The drawing under review shows one solid part. Ordinate dimensions are in mm from its lowest x, y, z. A direction names the side the tool comes from. Coordinates: 2 decimals unless noted, no trailing zeros. Order: outer loops, then holes, each group sorted by start corner. A loop starts at its lowest first (then second) coordinate and runs counter-clockwise, first axis right, second up.
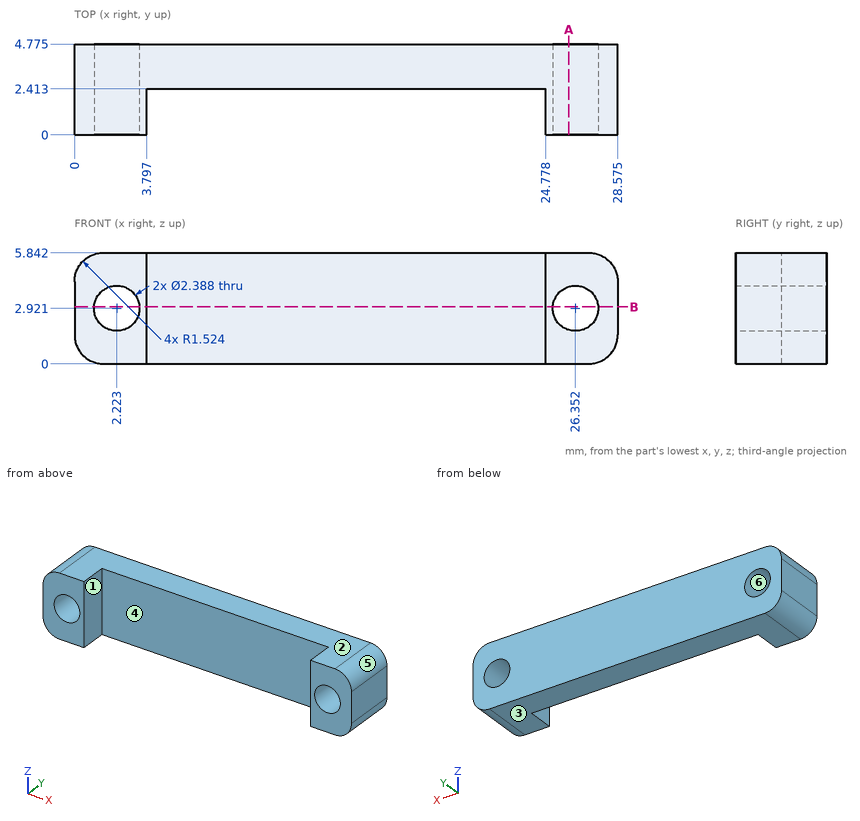
1. To check wall thickness, follow L1, parallel to X at y = 4, z = 2.85 (1 decimal); L2, parallel to X at y = 0.3, z = 1.45; L3, parallel to X at y = 3.4, z = 2 (1 decimal). State the ranges of each line that lie inside material, in increasing order.
Answer below:
L1: x = 0 to 1, 3.4 to 25.2, 27.5 to 28.6
L2: x = 0 to 3.8, 24.78 to 28.57
L3: x = 0 to 1.5, 3 to 25.6, 27.1 to 28.6
2. Machinability: for the marked faces 1 and 2, which of the approach directions +Z, -Z, +X, -X, +Y, -Y give a long, thin tool a straight path to every point of the face, cutting with its end or side? Answer none if there is none.
Answer below:
face 1: +Z, -Z, -Y
face 2: +Z, +X, -X, +Y, -Y
3. Clearance check with a flat-ended pin moving along its axis: pin 1 Ø1.4 at (x, z) = (26.35, 2.92) entering from -Y. State where the tip first meets the part, or that it passes through.
Answer below:
pin 1: passes through
4. The part is to be moulded in two halves that separate along Z. For the marked faces 3, 4, 5 and 6, say which applies: +Z half, -Z half, draft (parallel to the pull), parting line (faces both ways), or undercut.
Answer below:
face 3: -Z half
face 4: draft
face 5: +Z half
face 6: undercut
5. Take a section at A-A, the plane x = 26. Give the boundary of the cut face in (y, z) (1 decimal), plus the area to 3 significant figures.
Answer below:
outline: (0, 0) - (4.8, 0) - (4.8, 1.8) - (0, 1.8) - close; (0, 4.1) - (4.8, 4.1) - (4.8, 5.8) - (0, 5.8) - close
area: 17.0 mm2
6. Take a section at B-B, the plane z = 3. Give the number of separate pieces and of enclosed holes in the cut face.
Answer below:
separate pieces: 3
enclosed holes: 0
